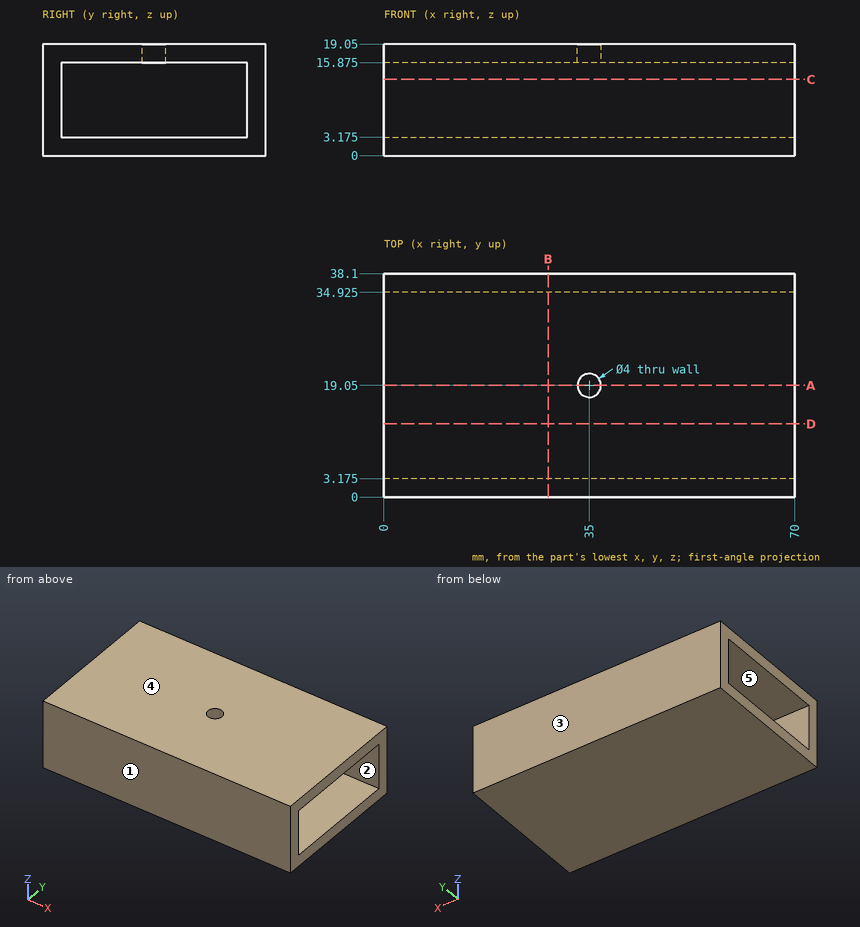
Input: dimensioned drawing with shaded views. Units: mm. Origin: part minimum x, y, z. A direction names the side the tool comes from. Give positions to 0.01 mm unless a question says otherwise; leave off trailing zeros. Loops run counter-clockwise (first coordinate to the right, second up) from the corner with the lowest first, then second, coordinate; pieces in that order, holes last. Notation, with made-up numbers: (84.25, 55.5) -> (101.25, 55.5) arc R7 ccw to (101.25, 66.5) -> close; hole circle Ø8 at (-40, 54). An arc over 180 degrees is marked (long way). Use a Markdown table: item, result. Add a question column.
1) Line query: line 1 along Y through (x, z) = (35, 16.95); line 2 along Z through (x, y) = (56, 28) (3 decimals); line 3 along Y through (x, z) = (14, 6) (3 decimals). Output: solid intervals per line, ascending. Write a range as [from, to].
2) First-contact query: pin 1 (2.5 mm diameter, centred on x = 35, y = 19.05, fed in from +Z) (3 decimals). Flat tip, straight axial feed; report the tip coordinate or a pass-through.
3) Section query B-B, the plane x = 28. Return the cut outline in (y, z) (3 decimals), then the cut area to 3 significant figures.
4) Pull-direction query (Y, two-part tool) for the marked faces 1, 2 and 3; classes: +Y half, -Y half, draft (parallel to the pull), parting line (faces both ways), or undercut.
5) Section query A-A, the plane y = 19.05. Return the cut outline in (x, z) (3 decimals), then the cut area to 3 significant figures.
6) Section query D-D, the plane y = 12.5. Return the cut outline in (x, z) (3 decimals).
7) Reachability of the marked faces 4 and 5 from +Z, -Z, +X, -X, +Y, -Y: full face, straight path, thin tool, end or side. Return the list, or none.
8) Section query C-C, the plane z = 13. Return the cut outline in (x, y) (3 decimals), then the cut area to 4 significant figures.
Numbers:
| question | item | result |
|---|---|---|
| 1 | line 1 | y = [0, 17.05], [21.05, 38.1] |
| 1 | line 2 | z = [0, 3.175], [15.875, 19.05] |
| 1 | line 3 | y = [0, 3.175], [34.925, 38.1] |
| 2 | pin 1 | stops at z = 3.175 |
| 3 | outline | (0, 0) -> (38.1, 0) -> (38.1, 19.05) -> (0, 19.05) -> close; hole (3.175, 3.175) -> (34.925, 3.175) -> (34.925, 15.875) -> (3.175, 15.875) -> close |
| 3 | area | 323 mm2 |
| 4 | face 1 | -Y half |
| 4 | face 2 | undercut |
| 4 | face 3 | +Y half |
| 5 | outline | (0, 0) -> (70, 0) -> (70, 3.175) -> (0, 3.175) -> close; (0, 15.875) -> (33, 15.875) -> (33, 19.05) -> (0, 19.05) -> close; (37, 15.875) -> (70, 15.875) -> (70, 19.05) -> (37, 19.05) -> close |
| 5 | area | 432 mm2 |
| 6 | outline | (0, 0) -> (70, 0) -> (70, 3.175) -> (0, 3.175) -> close; (0, 15.875) -> (70, 15.875) -> (70, 19.05) -> (0, 19.05) -> close |
| 7 | face 4 | +Z, +X, -X, +Y, -Y |
| 7 | face 5 | +X, -X |
| 8 | outline | (0, 0) -> (70, 0) -> (70, 3.175) -> (0, 3.175) -> close; (0, 34.925) -> (70, 34.925) -> (70, 38.1) -> (0, 38.1) -> close |
| 8 | area | 444.5 mm2 |
